from build123d import *

# Parameters (mm, degrees)
SKETCH10_R          = 101
BOSS_EXTRUDE5_DEPTH = 200
SKETCH5_R           = 101
BOSS_EXTRUDE6_DEPTH = 400
SKETCH11_R          = 100
CUT_EXTRUDE1_DEPTH  = 400
SKETCH12_R          = 100
CUT_EXTRUDE2_DEPTH  = 200


with BuildPart() as part:
    # Sketch10 → Boss-Extrude5 (new body)
    with BuildSketch(Plane(origin=(0, 0, 0), x_dir=(0, 0, -1), z_dir=(1, 0, 0))):
        with Locations((0, 200)):
            Circle(SKETCH10_R)
    extrude(amount=BOSS_EXTRUDE5_DEPTH)

    # Sketch5 → Boss-Extrude6 (add)
    with BuildSketch(Plane(origin=(0, 0, 0), x_dir=(1, 0, 0), z_dir=(0, 1, 0))):
        with Locations((200, 0)):
            Circle(SKETCH5_R)
    extrude(amount=BOSS_EXTRUDE6_DEPTH)

    # Sketch11 → Cut-Extrude1 (cut)
    with BuildSketch(Plane(origin=(0, 400, 0), x_dir=(1, 0, 0), z_dir=(0, 1, 0))):
        with Locations((200, 0)):
            Circle(SKETCH11_R)
    extrude(amount=-CUT_EXTRUDE1_DEPTH, mode=Mode.SUBTRACT)

    # Sketch12 → Cut-Extrude2 (cut)
    with BuildSketch(Plane.ZY):
        with Locations((0, 200)):
            Circle(SKETCH12_R)
    extrude(amount=-CUT_EXTRUDE2_DEPTH, mode=Mode.SUBTRACT)


solid = part.part
For this review, take the finished solid that the model builds, in its own axes (mm). A direction names the side the tool comes from. Give positions to 0.01 mm unless a question says otherwise; leave off trailing zeros. Order: outer loops, then holes, each group sorted by start corner. A loop starts at its lowest first (then second) coordinate and runs counter-clockwise, first axis right, second up. Notation, with made-up numbers: M -35,13.5 L 9,13.5 A25 cw 9,43.5 Z; hole C 74,61.5 d9. An arc over 180 degrees is marked long. Answer in a Markdown table with one row per item. Add a question column.
(1) Mouldability with a two-part tool opening along Z and no side actions: class faces 1 (the face through (76.378, 267.585, -73.704)), 2 (the face through (102, 400, -23)), 3 (the face through (76.38, 268.26, 74.44)) as +Z half, -Z half, draft (parallel to the pull), parting line (faces both ways), or undercut.
(2) Consider section B-B on x = 118. State the section outline as (y, z) points, and give its area (3 significant figures).
(3) For pin 1 (2 mm diameter, centred on x = 132, y = 357.5, fed in from +Z); pin 2 (10 mm diameter, centred on x = 151, y = 167.5, fed in from +Z); pin 3 (6 mm diameter, centred on y = 40.5, z = 14.5, fed in from +X), all flat-tipped, find the tip position at first contact; note any pin that passes through.
(4) Wall thickness on probe 1 along Y at (x, z) = (49.5, 0); probe 2 along Z at (x, y) = (135, 200); probe 3 along X at (y, z) = (84, -26): over which ranges is each line inside the solid? List them lowest first. Write a range as [from, to].
(5) For faces 4 (the face through (295.38, 202.8, -30.04)), 5 (the face through (293.3, 197.2, 38.68)), list the 3-axis set-ups (+Z, -Z, +X, -X, +Y, -Y) from which the entire face can be reached by the end or side of a thin tool; tool diameter is ignored.
(6) Consider section C-C on y = 200. State the section outline as (x, z) points, and give its area (3 significant figures).
(7) Consider section A-A on z = 0. State the section outline as (x, y) points.
(8) Consider section D-D on y = 354. State the section outline as (x, z) points.
Evaluation:
| question | item | result |
|---|---|---|
| 1 | face 1 | undercut |
| 1 | face 2 | draft |
| 1 | face 3 | parting line |
| 2 | outline | M 0,-58.97 L 118,-58.97 A101 ccw 282,-58.97 L 400,-58.97 L 400,-57.24 L 282,-57.24 A100 cw 118,-57.24 L 0,-57.24 Z; M 0,57.24 L 118,57.24 A100 cw 282,57.24 L 400,57.24 L 400,58.97 L 282,58.97 A101 ccw 118,58.97 L 0,58.97 Z |
| 2 | area | 1,200 mm^2 |
| 3 | pin 1 | stops at z = 75.58 |
| 3 | pin 2 | stops at z = 97.18 |
| 3 | pin 3 | stops at x = 300.34 |
| 4 | probe 1 | y = [99, 100], [300, 301] |
| 4 | probe 2 | z = [-101, -100], [100, 101] |
| 4 | probe 3 | x = [102.4, 103.44], [296.56, 297.6] |
| 5 | face 4 | +Y, -Y |
| 5 | face 5 | none |
| 6 | outline | M 0,-101 L 200,-101 A101 ccw 200,101 L 0,101 L 0,100 L 200,100 A100 cw 200,-100 L 0,-100 Z |
| 6 | area | 716 mm^2 |
| 7 | outline | M 0,99 L 99,99 L 99,0 L 100,0 L 100,100 L 0,100 Z; M 0,300 L 100,300 L 100,400 L 99,400 L 99,301 L 0,301 Z; M 300,0 L 301,0 L 301,400 L 300,400 Z |
| 8 | outline | C 200,0 d202; hole C 200,0 d200 |
